Read the model definition and answer for the solid it produces. Units are mm, in the model's axes. A direction names the side the tool comes from. Coordinates: 2 decimals unless noted, no trailing zeros. Write each loop counter-clockwise with the first axis right and the second up, starting at its lowest first coordinate (ties: lowest second). Pieces come first, ordered by that corner, then holes.
Item 1: Determine the mould class of faces 4 (the face through (52.16, 4.93, -17.7)), 5 (the face through (15, 33, -12)), 6 (the face through (59.465, 2.894, -6.576)) for opening direction X: released by +X, released by -X, zero draft, split by the parting line, or undercut.
Item 2: Section D-D (y = 24) is taken. Give the vertices of the cut face in (x, z), then the cut area to 3 significant figures.
Item 3: Section B-B (z = -40.64) is taken. Give the vertices of the cut face in (x, y).
Item 4: Section A-A (x = 53.19) is taken. Give the vertices of the cut face in (y, z), then the cut area to 3 significant figures.
Item 5: Each of these flat-tipped pins is pushed along its axis until it touches: P1, Ø6, axis at x = 22, y = 28, coming from the -Z side; P2, Ø2, axis at x = 58.5, y = 14.5, coming from the +Z side; P3, Ø3, axis at x = 53.19, z = -19.05, coming from the -Y side; P4, Ø4, axis at x = 45, z = -44, coming from the -Y side. Where does it stop, or does it pass through?
Item 6: A tool of negligible diameter and unlimited length cuts with its end or side. For faces 1 (the face through (59, 14, -41.931)), 2 (the face through (16, 10, -41)), 3 (the face through (59, 16.117, -36)), from which of +Z, -Z, +X, -X, +Y, -Y can it reach the whole face along a straight path? Write none if from no direction.
Item 7: Section C-C (x = 16.36) is taken. Give the vertices of the cut face in (y, z), then the cut area to 3 significant figures.
Item 8: Straight lines are drawn through the part: probe 1 along Z at (x, y) = (53, 4); probe 2 along Z at (x, y) = (16.5, 9); probe 3 along X at (y, z) = (4, -19.05). For each, find the intervals that lie inside material, in ascending order.
from build123d import *

# Parameters (mm, degrees)
SKETCH1_W           = 57
SKETCH1_H           = 44.5
BOSS_EXTRUDE1_DEPTH = 18
SKETCH2_R           = 2.314555985
SKETCH2_R_2         = 2.937250919
SKETCH2_W           = 10.945123542
SKETCH2_H           = 4.040448377
BOSS_EXTRUDE2_DEPTH = 5
SKETCH3_W           = 42
SKETCH3_H           = 24
BOSS_EXTRUDE3_DEPTH = 30
SKETCH4_W           = 15.5
SKETCH4_H           = 5
BOSS_EXTRUDE4_DEPTH = 20
SKETCH5_R           = 1.7
CUT_EXTRUDE1_DEPTH  = 10


with BuildPart() as part:
    # Sketch1 → Boss-Extrude1 (new body)
    with BuildSketch(Plane(origin=(0, 0, 0), x_dir=(1, 0, 0), z_dir=(0, 1, 0))):
        with Locations((28.5, 22.25)):
            Rectangle(SKETCH1_W, SKETCH1_H)
    extrude(amount=BOSS_EXTRUDE1_DEPTH)

    # Sketch2 → Boss-Extrude2 (add)
    with BuildSketch(Plane(origin=(57, 0, 0), x_dir=(0, 0, -1), z_dir=(1, 0, 0))):
        with Locations(Location((4.869948731, 4.458338777, 0), (0, 0, 180))):
            Circle(SKETCH2_R)
        with Locations(Location((10.656338694, 4.458338777, 0), (0, 0, 180))):
            Circle(SKETCH2_R_2)
        with Locations((36.458792801, 14.096318992)):
            Rectangle(SKETCH2_W, SKETCH2_H)
    extrude(amount=BOSS_EXTRUDE2_DEPTH)

    # Sketch3 → Boss-Extrude3 (add)
    with BuildSketch(Plane(origin=(0, 18, 0), x_dir=(1, 0, 0), z_dir=(0, 1, 0))):
        with Locations((36, 12)):
            Rectangle(SKETCH3_W, SKETCH3_H)
    extrude(amount=BOSS_EXTRUDE3_DEPTH)

    # Sketch4 → Boss-Extrude4 (add)
    with BuildSketch(Plane(origin=(0, 0, -44.5), x_dir=(-1, 0, 0), z_dir=(0, 0, -1))):
        with Locations((-10.25, 14)):
            Rectangle(SKETCH4_W, SKETCH4_H)
    extrude(amount=BOSS_EXTRUDE4_DEPTH)

    # Sketch5 → Cut-Extrude1 (cut)
    with BuildSketch(Plane.XZ):
        with Locations(Location((3.66, -3.81, 0), (0, 0, 270))):
            Circle(SKETCH5_R)
        with Locations(Location((16.36, -40.64, 0), (0, 0, 270))):
            Circle(SKETCH5_R)
        with Locations(Location((53.19, -19.05, 0), (0, 0, 270))):
            Circle(SKETCH5_R)
    extrude(amount=-CUT_EXTRUDE1_DEPTH, mode=Mode.SUBTRACT)


solid = part.part
Established:
1. face 4: undercut
1. face 5: released by -X
1. face 6: zero draft
2. outline: (15, -24) - (57, -24) - (57, 0) - (15, 0) - close
2. area: 1,010 mm2
3. outline: (0, 0) - (14.66, 0) - (14.66, 10) - (18.06, 10) - (18.06, 0) - (57, 0) - (57, 12.08) - (62, 12.08) - (62, 16.12) - (57, 16.12) - (57, 18) - (0, 18) - close
4. outline: (0, -44.5) - (18, -44.5) - (18, -24) - (48, -24) - (48, 0) - (0, 0) - (0, -17.35) - (10, -17.35) - (10, -20.75) - (0, -20.75) - close
4. area: 1,490 mm2
5. P1: stops at z = -24
5. P2: stops at z = -30.99
5. P3: stops at y = 10
5. P4: stops at y = 0
6. face 1: -Z, +X, +Y, -Y
6. face 2: -Y
6. face 3: +Z, -Z, +X, +Y
7. outline: (0, -44.5) - (11.5, -44.5) - (11.5, -64.5) - (16.5, -64.5) - (16.5, -44.5) - (18, -44.5) - (18, -24) - (48, -24) - (48, 0) - (0, 0) - (0, -38.94) - (10, -38.94) - (10, -42.34) - (0, -42.34) - close
7. area: 1,590 mm2
8. probe 1: z = -44.5 to -20.74, -17.36 to 0
8. probe 2: z = -44.5 to -42.33, -38.95 to 0
8. probe 3: x = 0 to 51.49, 54.89 to 57
